Can you work these out from the drawing? Everything is in mm from the part's minimum corner. Give positions to 0.01 mm unless a question says otherwise; leave off trailing zeros. Write each loop counter-clockwise with the first axis right and the second up, starting at its lowest first coordinate (ties: lowest second). Pieces come first, ordered by that corner, then holes. Notation, with made-up numbers: (51, 38) -> (100, 38) arc R15 cw to (100, 60) -> close; hole circle Ø5 at (-39, 80.5). An arc over 180 degrees is marked (long way). Answer as CSV lines item,"result". Start each with the question number.
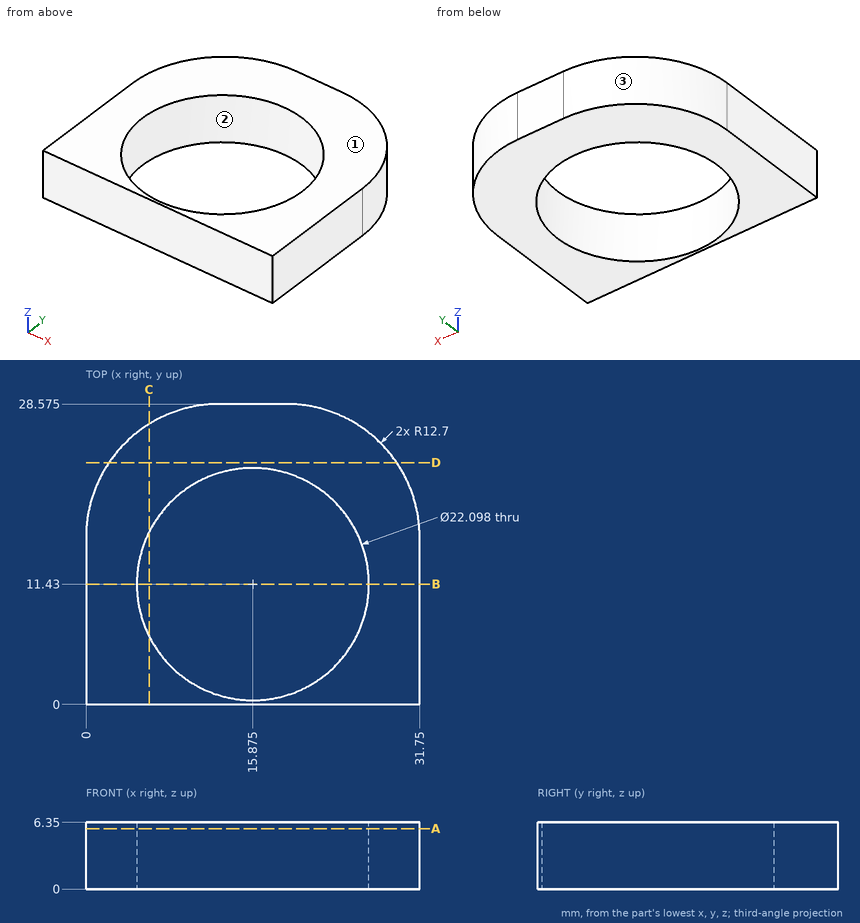
Item 1: We'd pull the mould along Y, two halves only. Please class the marked faces 1, 2 and 3: released by +Y, released by -Y, zero draft, split by the parting line, or undercut.
Item 2: I'm going to push a flat-ended pin straight in: pin 1 (1.5 mm diameter, centred on y = 20, z = 1.5, fed in from -X). Where does the tip first touch, or does it pass through?
Item 3: If I drill on line 1 (X direction, y = 18.25, z = 0.75); line 2 (Y direction, x = 15.5, z = 5.75) (3 decimals); line 3 (X direction, y = 6.25, z = 6), over which ranges is the centre line in solid material (lowest first)? Write a range as [from, to].
Item 4: If we section it at D-D (y = 23): Please give me the cut outline in (x, z), and give its area (3 significant figures).
Item 5: If we section it at B-B (y = 11.43): Please give me the cut outline in (x, z), and give its area (3 significant figures).
Item 6: If we section it at C-C (x = 6): Please give me the cut outline in (y, z), and give its area (3 significant figures).
Item 7: If we section it at A-A (z = 5.75): Please give me the cut outline in (x, y) (3 decimals).
Final values:
1,face 1,"zero draft"
1,face 2,"undercut"
1,face 3,"released by +Y"
2,pin 1,"x = 0.46"
3,line 1,"[0.22, 7.18], [24.57, 31.53]"
3,line 2,"[0, 0.387], [22.473, 28.575]"
3,line 3,"[0, 6.12], [25.63, 31.75]"
4,outline,"(2.19, 0) -> (29.56, 0) -> (29.56, 6.35) -> (2.19, 6.35) -> close"
4,area,"174 mm2"
5,outline,"(0, 0) -> (4.83, 0) -> (4.83, 6.35) -> (0, 6.35) -> close; (26.92, 0) -> (31.75, 0) -> (31.75, 6.35) -> (26.92, 6.35) -> close"
5,area,"61.3 mm2"
6,outline,"(0, 0) -> (6.47, 0) -> (6.47, 6.35) -> (0, 6.35) -> close; (16.39, 0) -> (26.66, 0) -> (26.66, 6.35) -> (16.39, 6.35) -> close"
6,area,"106 mm2"
7,outline,"(0, 0) -> (31.75, 0) -> (31.75, 15.875) arc R12.7 ccw to (19.05, 28.575) -> (12.7, 28.575) arc R12.7 ccw to (0, 15.875) -> close; hole circle Ø22.098 at (15.875, 11.43)"
